Verification items for the finished model (mm, model axes). A direction names the side the tool comes from. Coordinates: 2 decimals unless noted, no trailing zeros. Order: outer loops, then holes, each group sorted by start corner. A loop starts at its lowest first (then second) coordinate and runs counter-clockwise, first axis right, second up.
Q1. Cross-section at D-D, the plane y = -8.75. Record the boundary of the cut face in (x, z).
Q2. Depth check by flat-ended pin: P1, Ø2, axis at y = -4.5, z = 46, coming from the -X side; P2, Ø5, axis at x = 8.5, z = 13.5, coming from the -Y side; P3, Ø4.5, axis at y = -4.5, z = 9, coming from the -X side; P4, Ø2, axis at y = -8.5, z = 26, coming from the +X side. Enter the tip coordinate at first touch or a pass-through.
Q3. Cross-section at A-A, the plane z = 13.75. Record the boundary of the cut face in (x, y).
Q4. Thickness scan on line 1 (Z direction, x = 1.5, y = -4.5); line 2 (X direction, y = 1.95, z = 13.75); line 3 (Z direction, x = 9.75, y = -3). Record the ranges inside material, lowest first.
Q5. Set-up check for faces 1 (the flat face through (7, 0.5, 41.3)), 2 (the flat face through (5, -3, 55)), 3 (the flat face through (9, 0, 27)): record each of +Z, -Z, +X, -X, +Y, -Y from which the full face is reachable in a straight line by a thin tool's end or side.
Q6. Cross-section at B-B, the plane z = 33. Record the boundary of the cut face in (x, y), and give its area (3 significant figures).
Q7. Draft check along Y on faces 4 (the cylindrical face through (9.423, -0.301, 3.285)), 5 (the flat face through (8.479, 0.493, 11.164)), 6 (the cylindrical face through (1.479, -4.285, 47.636)). Enter one of: pulls with the +Y half, pulls with the -Y half, needs draft (parallel to the pull), parting line crosses it, or undercut.
Q8. Cross-section at C-C, the plane x = 4.5. Record the boundary of the cut face in (y, z) (3 decimals).
from build123d import *

# Parameters (mm, degrees)
ESQUISSE2_W             = 15
ESQUISSE2_H             = 3
BOSS_EXTRU_1_DEPTH      = 55
BOSS_EXTRU_2_DEPTH      = 3
BOSS_EXTRU_3_DEPTH      = 3
CONG_1_R                = 3
CONG_2_R                = 1
CONG_3_START            = 4
CONG_3_3_DEPTH          = 47
CONG_3_START_2          = -1
CONG_3_4_DEPTH          = 57
ENL_V_MAT_EXTRU_1_REACH = 61.211
ESQUISSE5_R             = 1.65
ENL_V_MAT_EXTRU_2_DEPTH = 1
ESQUISSE8_R             = 1.65
ENL_V_MAT_EXTRU_3_DEPTH = 59.472215766


with BuildPart() as part:
    # Esquisse2 → Boss.-Extru.1 (new body)
    with BuildSketch(Plane.XY):
        with BuildLine():
            Line((3, 0), (0, 0))
            Line((0, 0), (0, -12))
            ThreePointArc((0, -12), (0.292893219, -12.707106781), (1, -13))
            Line((1, -13), (3, -13))
            Line((3, -13), (3, 0))
        make_face()
        with Locations((7.5, 1.5)):
            Rectangle(ESQUISSE2_W, ESQUISSE2_H)
    extrude(amount=BOSS_EXTRU_1_DEPTH)

    # Esquisse3 → Boss.-Extru.2 (add)
    with BuildSketch(Plane(origin=(3, 0, 55), x_dir=(-1, 0, 0), z_dir=(0, 0, -1))):
        Polygon((-12, 0), (0, -13), (0, 0), align=None)
    extrude(amount=BOSS_EXTRU_2_DEPTH)

    # Esquisse4 → Boss.-Extru.3 (add)
    with BuildSketch(Plane(origin=(3, 0, 0), x_dir=(-1, 0, 0), z_dir=(0, 0, -1))):
        Polygon((0, 0), (-12, 0), (0, -13), align=None)
    extrude(amount=-BOSS_EXTRU_3_DEPTH)

    # Congé1
    cong_1_edges = [part.edges().sort_by_distance(p)[0] for p in [
        (15, 1.5, 0),
        (15, 1.5, 55),
    ]]
    fillet(cong_1_edges, radius=CONG_1_R)

    # Congé2
    # the kernel refuses this fillet: 1 mm, written as the material it adds along each edge
    with BuildSketch(Plane(origin=(4, -1, 4), x_dir=(0, 1, 0), z_dir=(-1, 0, 0))) as cong_2_piece_1_section:
        Polygon((0, 0), (CONG_2_R, 0), (CONG_2_R, CONG_2_R), (0, CONG_2_R), align=None)
    cong_2_piece_1 = extrude(amount=CONG_2_R, mode=Mode.PRIVATE)
    cong_2_piece_1 = cong_2_piece_1 - Plane(origin=(4, -1, 4), x_dir=(0, -0.7071067811865475, 0.7071067811865475), z_dir=(-1, 0, 0)) * Sphere(CONG_2_R, mode=Mode.PRIVATE)
    add(cong_2_piece_1)
    with BuildSketch(Plane(origin=(4, -1, 51), x_dir=(0, 1, 0), z_dir=(-1, 0, 0))) as cong_2_piece_2_section:
        Polygon((0, 0), (CONG_2_R, 0), (CONG_2_R, -CONG_2_R), (0, -CONG_2_R), align=None)
    cong_2_piece_2 = extrude(amount=CONG_2_R, mode=Mode.PRIVATE)
    cong_2_piece_2 = cong_2_piece_2 - Plane(origin=(4, -1, 51), x_dir=(0, -0.7071067811865475, -0.7071067811865475), z_dir=(-1, 0, 0)) * Sphere(CONG_2_R, mode=Mode.PRIVATE)
    add(cong_2_piece_2)
    with BuildSketch(Plane(origin=(3, 0, 4), x_dir=(0, -1, 0), z_dir=(0, 0, 1))) as cong_2_piece_3:
        with BuildLine():
            CenterArc((CONG_2_R, CONG_2_R), CONG_2_R, 180, 90)
            Line((0, CONG_2_R), (0, 0))
            Line((0, 0), (CONG_2_R, 0))
        make_face()
    extrude(amount=47)
    with BuildSketch(Plane(origin=(4, 0, 52), x_dir=(0, 0, -1), z_dir=(1, 0, 0))) as cong_2_piece_4_section:
        with BuildLine():
            CenterArc((CONG_2_R, -CONG_2_R), CONG_2_R, 90, 90)
            Line((0, -CONG_2_R), (0, 0))
            Line((0, 0), (CONG_2_R, 0))
        make_face()
    cong_2_piece_4 = extrude(amount=11, mode=Mode.PRIVATE)
    cong_2_piece_4 = split(cong_2_piece_4, bisect_by=Plane(origin=(9.939297125, -5.482428115, 52), z_dir=(-0.7348034446274879, 0.6782801027330657, 0)), keep=Keep.TOP, mode=Mode.PRIVATE)
    add(cong_2_piece_4)
    with BuildSketch(Plane(origin=(3, -13, 52), x_dir=(0, 0, -1), z_dir=(0, 1, 0))) as cong_2_piece_5_section:
        with BuildLine():
            CenterArc((CONG_2_R, -CONG_2_R), CONG_2_R, 90, 90)
            Line((0, -CONG_2_R), (0, 0))
            Line((0, 0), (CONG_2_R, 0))
        make_face()
    cong_2_piece_5 = extrude(amount=12, mode=Mode.PRIVATE)
    cong_2_piece_5 = split(cong_2_piece_5, bisect_by=Plane(origin=(3, -13, 52), z_dir=(-0.7348034446274879, 0.6782801027330657, 0)), keep=Keep.TOP, mode=Mode.PRIVATE)
    add(cong_2_piece_5)
    with BuildSketch(Plane(origin=(3, -13, 3), x_dir=(1, 0, 0), z_dir=(0, 1, 0))) as cong_2_piece_6_section:
        with BuildLine():
            CenterArc((CONG_2_R, -CONG_2_R), CONG_2_R, 90, 90)
            Line((0, -CONG_2_R), (0, 0))
            Line((0, 0), (CONG_2_R, 0))
        make_face()
    cong_2_piece_6 = extrude(amount=12, mode=Mode.PRIVATE)
    cong_2_piece_6 = split(cong_2_piece_6, bisect_by=Plane(origin=(3, -13, 3), z_dir=(-0.7348034446274879, 0.6782801027330657, 0)), keep=Keep.TOP, mode=Mode.PRIVATE)
    add(cong_2_piece_6)
    with BuildSketch(Plane(origin=(4, 0, 3), x_dir=(0, -1, 0), z_dir=(1, 0, 0))) as cong_2_piece_7_section:
        with BuildLine():
            CenterArc((CONG_2_R, -CONG_2_R), CONG_2_R, 90, 90)
            Line((0, -CONG_2_R), (0, 0))
            Line((0, 0), (CONG_2_R, 0))
        make_face()
    cong_2_piece_7 = extrude(amount=11, mode=Mode.PRIVATE)
    cong_2_piece_7 = split(cong_2_piece_7, bisect_by=Plane(origin=(9.939297125, -5.482428115, 3), z_dir=(-0.7348034446274879, 0.6782801027330657, 0)), keep=Keep.TOP, mode=Mode.PRIVATE)
    add(cong_2_piece_7)

    # Congé3: read off the stored shape, not the designer's step
    # Congé3 outline → Congé3 (revolve, cut)
    with BuildSketch(Plane(origin=(4, 0, 51), x_dir=(1, 0, 0), z_dir=(0, 0, 1))):
        with BuildLine():
            ThreePointArc((2, -13), (1.292893219, -12.707106781), (1, -12))
            Line((1, -12), (1, -13))
            Line((1, -13), (2, -13))
        make_face()
    revolve(axis=Axis((4, 0, 51), (0, 1, 0)), mode=Mode.SUBTRACT)

    # Cong_3 2 outline → Cong_3 2 (revolve, cut)
    with BuildSketch(Plane(origin=(4, 0, 4), x_dir=(1, 0, 0), z_dir=(0, 0, 1))):
        with BuildLine():
            ThreePointArc((2, -13), (1.292893219, -12.707106781), (1, -12))
            Line((1, -12), (1, -13))
            Line((1, -13), (2, -13))
        make_face()
    revolve(axis=Axis((4, 0, 4), (0, 1, 0)), mode=Mode.SUBTRACT)

    # Cong_3 3 outline → Cong_3 3 (cut)
    with BuildSketch(Plane.XY.offset(CONG_3_START)):
        with BuildLine():
            Line((2, -13), (3, -13))
            Line((3, -13), (3, -12))
            ThreePointArc((3, -12), (2.707106781, -12.707106781), (2, -13))
        make_face()
    extrude(amount=CONG_3_3_DEPTH, mode=Mode.SUBTRACT)

    # Cong_3 4 outline → Cong_3 4 (cut)
    with BuildSketch(Plane.XY.offset(CONG_3_START_2)):
        with BuildLine():
            Line((2.562168768, -13), (3, -13))
            Line((3, -13), (3.296972213, -12.678280103))
            ThreePointArc((3.296972213, -12.678280103), (2.963242263, -12.916045878), (2.562168768, -13))
        make_face()
    extrude(amount=CONG_3_4_DEPTH, mode=Mode.SUBTRACT)

    # Esquisse5 → Enlèv. mat.-Extru.1 (cut, up to next)
    with BuildSketch(Plane(origin=(0, 3, 0), x_dir=(1, 0, 0), z_dir=(0, 1, 0)), mode=Mode.PRIVATE) as enl_v_mat_extru_1_sk1:
        with Locations(Location((10, -41.25, 0), (0, 0, 270))):
            Circle(ESQUISSE5_R)
    enl_v_mat_extru_1_tool1 = extrude(enl_v_mat_extru_1_sk1.sketch, amount=-ENL_V_MAT_EXTRU_1_REACH, mode=Mode.PRIVATE) & part.part
    # Esquisse5 → Enlèv. mat.-Extru.1 (cut, up to next)
    with BuildSketch(Plane(origin=(0, 3, 0), x_dir=(1, 0, 0), z_dir=(0, 1, 0)), mode=Mode.PRIVATE) as enl_v_mat_extru_1_sk2:
        with Locations(Location((10, -13.75, 0), (0, 0, 270))):
            Circle(ESQUISSE5_R)
    enl_v_mat_extru_1_tool2 = extrude(enl_v_mat_extru_1_sk2.sketch, amount=-ENL_V_MAT_EXTRU_1_REACH, mode=Mode.PRIVATE) & part.part
    add(enl_v_mat_extru_1_tool1.solids().sort_by_distance((10, 3, 41.25))[0], mode=Mode.SUBTRACT)
    add(enl_v_mat_extru_1_tool2.solids().sort_by_distance((10, 3, 13.75))[0], mode=Mode.SUBTRACT)

    # Esquisse7 → Enlèv. mat.-Extru.2 (cut)
    with BuildSketch(Plane(origin=(0, 0, 0), x_dir=(-1, 0, 0), z_dir=(0, -1, 0))):
        Polygon((-10, -37.785898385), (-13, -39.517949192), (-13, -42.982050808), (-10, -44.714101615), (-7, -42.982050808), (-7, -39.517949192), align=None)
        Polygon((-10, -10.285898385), (-13, -12.017949192), (-13, -15.482050808), (-10, -17.214101615), (-7, -15.482050808), (-7, -12.017949192), align=None)
    extrude(amount=-ENL_V_MAT_EXTRU_2_DEPTH, mode=Mode.SUBTRACT)

    # Esquisse8 → Enlèv. mat.-Extru.3 (cut, through all)
    with BuildSketch(Plane.ZY):
        with Locations(Location((46, -4.5, 0), (0, 0, 270))):
            Circle(ESQUISSE8_R)
        with Locations(Location((9, -4.5, 0), (0, 0, 270))):
            Circle(ESQUISSE8_R)
    extrude(amount=-ENL_V_MAT_EXTRU_3_DEPTH, mode=Mode.SUBTRACT)


solid = part.part
Check values:
1. outline: (0, 0) - (6.92, 0) - (6.92, 3) - (4, 3) arc R1 cw to (3, 4) - (3, 51) arc R1 cw to (4, 52) - (6.92, 52) - (6.92, 55) - (0, 55) - close
2. P1: passes through
2. P2: stops at y = 0
2. P3: stops at x = 0
2. P4: stops at x = 3
3. outline: (0, -12) arc R1 ccw to (1, -13) - (2, -13) arc R1 ccw to (3, -12) - (3, -1) arc R1 cw to (4, 0) - (7, 0) - (7, 1) - (8.35, 1) - (8.35, 3) - (0, 3) - close; (11.65, 1) - (13, 1) - (13, 0) - (15, 0) - (15, 3) - (11.65, 3) - close
4. line 1: z = 0 to 7.35, 10.65 to 44.35, 47.65 to 55
4. line 2: x = 0 to 8.35, 11.65 to 15
4. line 3: z = 0 to 3, 52 to 55
5. face 1: -Y
5. face 2: +Z, +X, -X, +Y, -Y
5. face 3: +X, -Y
6. outline: (0, -12) arc R1 ccw to (1, -13) - (2, -13) arc R1 ccw to (3, -12) - (3, -1) arc R1 cw to (4, 0) - (15, 0) - (15, 3) - (0, 3) - close
6. area: 83.8 mm2
7. face 4: pulls with the -Y half
7. face 5: needs draft
7. face 6: undercut
8. outline: (-11.375, 0) - (3, 0) - (3, 55) - (-11.375, 55) - (-11.375, 52) - (-1, 52) arc R1 cw to (0, 51) - (0, 4) arc R1 cw to (-1, 3) - (-11.375, 3) - close
